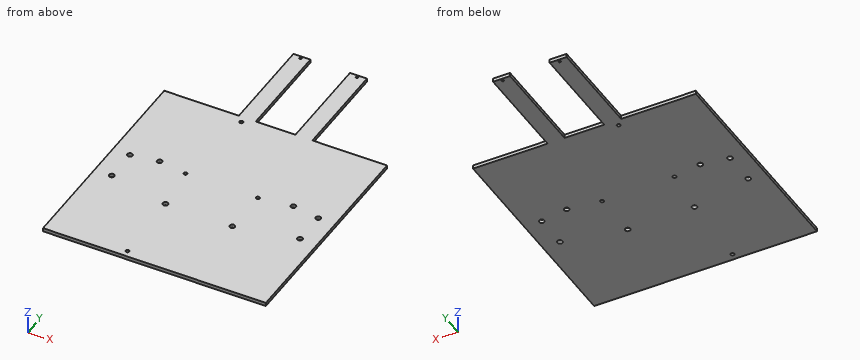
from build123d import *

# Parameters (mm, degrees)
F0_W     = 51.8
F0_H     = 10
F0_W_2   = 15.24
F0_H_2   = 34.925
F0_R     = 2.3114
F0_R_2   = 1.05
F0_R_3   = 1.5875
F0_W_3   = 9.38
F1_DEPTH = 3.175
F2_DEPTH = 90


# Not quite as in the source:
# - a length typed as a fraction of an inch, garbled in the dataset ("3 / 203.2 mm" for 3/8 in), is restored
# - a feature names something its author has since deleted; it is built from what else it names


with BuildPart() as f1:
    # F0 (on Top) → F1 (new body)
    with BuildSketch(Plane.XY):
        Polygon((42.4, -100), (100, -100), (100, -75.075), (48.2, -75.075), (48.2, -65.075), (33.02, -65.075), (33.02, -100), align=None)
        with Locations((74.1, -70.075)):
            Rectangle(F0_W, F0_H)
        Polygon((33.02, -140), (33.02, -100), (17.78, -100), (17.78, -140), (17.78, -190), (25.4, -190), (33.02, -190), align=None)
        with BuildLine():
            ThreePointArc((26.45, -187.7), (26.1424621202, -188.4424621202), (25.4, -188.75))
            ThreePointArc((25.4, -188.75), (24.6575378798, -186.9575378798), (26.45, -187.7))
        make_face(mode=Mode.SUBTRACT)
        with Locations((25.4, -82.5375)):
            Rectangle(F0_W_2, F0_H_2)
        with Locations((74.1, -60.075)):
            Rectangle(F0_W, F0_H)
        Polygon((0, -100), (17.78, -100), (17.78, -65.075), (-17.78, -65.075), (-17.78, -100), align=None)
        Polygon((17.78, -65.075), (33.02, -65.075), (48.2, -65.075), (48.2, -55.075), (-48.2, -55.075), (-48.2, -65.075), (-33.02, -65.075), (-17.78, -65.075), align=None)
        with BuildLine():
            Line((48.2, -55.075), (100, -55.075))
            Line((100, -55.075), (100, -26.575))
            Line((100, -26.575), (32.3114, -26.575))
            ThreePointArc((32.3114, -26.575), (30, -28.8864), (27.6886, -26.575))
            Line((27.6886, -26.575), (0, -26.575))
            Line((0, -26.575), (-27.6886, -26.575))
            ThreePointArc((-27.6886, -26.575), (-30, -28.8864), (-32.3114, -26.575))
            Line((-32.3114, -26.575), (-100, -26.575))
            Line((-100, -26.575), (-100, -55.075))
            Line((-100, -55.075), (-48.2, -55.075))
            Line((-48.2, -55.075), (48.2, -55.075))
        make_face()
        with BuildLine():
            Line((32.3114, -26.575), (100, -26.575))
            Line((100, -26.575), (100, 0))
            Line((100, 0), (0, 0))
            Line((0, 0), (0, -10.4469014332))
            Line((0, -10.4469014332), (0, -26.575))
            Line((0, -26.575), (27.6886, -26.575))
            ThreePointArc((27.6886, -26.575), (30, -24.2636), (32.3114, -26.575))
        make_face()
        with Locations((84.5, -15)):
            Circle(F0_R, mode=Mode.SUBTRACT)
        Polygon((-17.78, -140), (-17.78, -100), (-27.462, -100), (-33.02, -100), (-33.02, -140), (-33.02, -190), (-25.4, -190), (-17.78, -190), align=None)
        with BuildLine():
            ThreePointArc((-24.35, -187.7), (-24.6575378798, -188.4424621202), (-25.4, -188.75))
            ThreePointArc((-25.4, -188.75), (-26.1424621202, -186.9575378798), (-24.35, -187.7))
        make_face(mode=Mode.SUBTRACT)
        with Locations((-25.4, -137.7)):
            Circle(F0_R_2, mode=Mode.SUBTRACT)
        Polygon((-27.462, -100), (-17.78, -100), (-17.78, -65.075), (-33.02, -65.075), (-33.02, -100), align=None)
        with BuildLine():
            ThreePointArc((-25.8745, -93.912), (-26.3394679849, -95.0345320151), (-27.462, -95.4995))
            ThreePointArc((-27.462, -95.4995), (-29.0495, -93.912), (-27.462, -92.3245))
            ThreePointArc((-27.462, -92.3245), (-26.3394679849, -92.7894679849), (-25.8745, -93.912))
        make_face(mode=Mode.SUBTRACT)
        with BuildLine():
            Line((0, 0), (100, 0))
            Line((100, 0), (100, 55.075))
            Line((100, 55.075), (48.2, 55.075))
            Line((48.2, 55.075), (48.2, 65.075))
            Line((48.2, 65.075), (42.4, 65.075))
            Line((42.4, 65.075), (42.4, 18.9709383994))
            Line((42.4, 18.9709383994), (42.4, 9.75))
            Line((42.4, 9.75), (30.355, 9.75))
            Line((30.355, 9.75), (-42.4, 9.75))
            Line((-42.4, 9.75), (-42.4, 65.075))
            Line((-42.4, 65.075), (-48.2, 65.075))
            Line((-48.2, 65.075), (-48.2, 55.075))
            Line((-48.2, 55.075), (-100, 55.075))
            Line((-100, 55.075), (-100, 0))
            Line((-100, 0), (-100, -26.575))
            Line((-100, -26.575), (-32.3114, -26.575))
            ThreePointArc((-32.3114, -26.575), (-30, -24.2636), (-27.6886, -26.575))
            Line((-27.6886, -26.575), (0, -26.575))
            Line((0, -26.575), (0, -10.4469014332))
            Line((0, -10.4469014332), (0, 0))
        make_face()
        with BuildLine():
            ThreePointArc((-82.1886, -15), (-86.134406614, -16.634406614), (-84.5, -12.6886))
            ThreePointArc((-84.5, -12.6886), (-82.865593386, -13.365593386), (-82.1886, -15))
        make_face(mode=Mode.SUBTRACT)
        with BuildLine():
            ThreePointArc((-82.1886, 15), (-82.865593386, 13.365593386), (-84.5, 12.6886))
            ThreePointArc((-84.5, 12.6886), (-86.134406614, 16.634406614), (-82.1886, 15))
        make_face(mode=Mode.SUBTRACT)
        with Locations((-60, 18.9709383994)):
            Circle(F0_R, mode=Mode.SUBTRACT)
        with BuildLine():
            ThreePointArc((62.3114, 18.9709383994), (60, 16.6595383994), (57.6886, 18.9709383994))
            ThreePointArc((57.6886, 18.9709383994), (60, 21.2823383994), (62.3114, 18.9709383994))
        make_face(mode=Mode.SUBTRACT)
        with Locations((84.5, 15)):
            Circle(F0_R, mode=Mode.SUBTRACT)
        with Locations((-74.1, -60.075)):
            Rectangle(F0_W, F0_H)
        Polygon((-33.02, -100), (-33.02, -65.075), (-48.2, -65.075), (-48.2, -75.075), (-100, -75.075), (-100, -100), (-42.4, -100), align=None)
        with Locations((74.1, 60.075)):
            Rectangle(F0_W, F0_H)
        with Locations((-74.1, -70.075)):
            Rectangle(F0_W, F0_H)
        with Locations((74.1, 70.075)):
            Rectangle(F0_W, F0_H)
        Polygon((48.2, 75.075), (100, 75.075), (100, 100), (42.4, 100), (42.4, 65.075), (48.2, 65.075), align=None)
        Polygon((42.4, 18.9709383994), (42.4, 65.075), (42.4, 100), (33.02, 100), (17.78, 100), (0, 100), (-17.78, 100), (-27.462, 100), (-33.02, 100), (-33.02, 65.075), (-42.4, 65.075), (-42.4, 9.75), (30.355, 9.75), (42.4, 9.75), align=None)
        with Locations((-34.645, 14.954)):
            Circle(F0_R_3, mode=Mode.SUBTRACT)
        with BuildLine():
            ThreePointArc((-27.462, 92.3245), (-29.0495, 93.912), (-27.462, 95.4995))
            ThreePointArc((-27.462, 95.4995), (-26.3394679849, 95.0345320151), (-25.8745, 93.912))
            ThreePointArc((-25.8745, 93.912), (-26.3394679849, 92.7894679849), (-27.462, 92.3245))
        make_face(mode=Mode.SUBTRACT)
        with BuildLine():
            ThreePointArc((31.9425, 14.954), (31.4775320151, 13.8314679849), (30.355, 13.3665))
            ThreePointArc((30.355, 13.3665), (29.2324679849, 13.8314679849), (28.7675, 14.954))
            ThreePointArc((28.7675, 14.954), (30.355, 16.5415), (31.9425, 14.954))
        make_face(mode=Mode.SUBTRACT)
        with Locations((-74.1, 60.075)):
            Rectangle(F0_W, F0_H)
        with Locations((-74.1, 70.075)):
            Rectangle(F0_W, F0_H)
        Polygon((17.78, 100), (33.02, 100), (33.02, 140), (33.02, 190), (25.4, 190), (17.78, 190), (17.78, 140), align=None)
        with BuildLine():
            ThreePointArc((26.45, 187.7), (24.6575378798, 186.9575378798), (25.4, 188.75))
            ThreePointArc((25.4, 188.75), (26.1424621202, 188.4424621202), (26.45, 187.7))
        make_face(mode=Mode.SUBTRACT)
        Polygon((-100, 100), (-100, 75.075), (-48.2, 75.075), (-48.2, 65.075), (-42.4, 65.075), (-42.4, 100), align=None)
        with Locations((-37.71, 82.5375)):
            Rectangle(F0_W_3, F0_H_2)
        Polygon((-27.462, 100), (-17.78, 100), (-17.78, 140), (-17.78, 190), (-25.4, 190), (-33.02, 190), (-33.02, 140), (-33.02, 100), align=None)
        with BuildLine():
            ThreePointArc((-24.35, 187.7), (-26.1424621202, 186.9575378798), (-25.4, 188.75))
            ThreePointArc((-25.4, 188.75), (-24.6575378798, 188.4424621202), (-24.35, 187.7))
        make_face(mode=Mode.SUBTRACT)
        with Locations((-25.4, -137.7)):
            Circle(F0_R_2)
    extrude(amount=F1_DEPTH)

    # F2 (cut): faces of the model
    f2_faces = [f1.faces().sort_by_distance(p)[0] for p in [
        (25.4, -190, 1.5875),
        (-25.4, -190, 1.5875),
    ]]
    extrude(f2_faces, amount=-F2_DEPTH, mode=Mode.SUBTRACT)


solid = f1.part
The listing builds one solid part. Answer for the finished solid, in the listing's coordinates (mm). Coordinates: 2 decimals unless noted, no trailing zeros. Write each loop counter-clockwise with the first axis right and the second up, starting at its lowest first coordinate (ties: lowest second). Pieces come first, ordered by that corner, then holes. Notation, with made-up numbers: M 53.25,86 L 62.25,86 A23 cw 62.25,118 Z; hole C 82.25,-26.5 d6. An arc over 180 degrees is marked long. Put each result on its own line as item: value. Start each with the question number.
1. Consider line 1 (X direction, y = 187.7, z = 0.75); line 2 (Y direction, x = 84.5, z = 2.1); line 3 (X direction, y = -28.5, z = 2.3). Determine where each line is inside the solid, lowest interval first. Write a range as from..to.
2. Flat-ended cylindrical pins translate along their axes: P1, Ø3, axis at x = 84.5, y = 15, coming from the +Z side; P2, Ø2.5, axis at x = -25.4, y = 187.7, coming from the +Z side (3 decimals); P3, Ø1, axis at y = 148.5, z = 1, coming from the -X side. Find the tip coordinate at first contact, or state that the pin passes through.
3. A cutting plane is placed at C-C on z = 1.1. Count the separate pieces of the cut face and the enclosed holes in it, then the cut area to 3 significant figures.
4. A cutting plane is placed at B-B on x = -44. Write down the section's boundary in (y, z) (3 decimals).
5. A cutting plane is placed at A-A on y = 154. Write down the section's boundary in (x, z) (3 decimals).
Resolved:
1. line 1: x = -33.02..-26.45, -24.35..-17.78, 17.78..24.35, 26.45..33.02
1. line 2: y = -100..-17.31, -12.69..12.69, 17.31..100
1. line 3: x = -100..-31.28, -28.72..28.72, 31.28..100
2. P1: passes through
2. P2: stops at z = 3.175
2. P3: stops at x = -33.02
3. separate pieces: 1
3. enclosed holes: 14
3. area: 42,600 mm2
4. outline: M -100,0 L 100,0 L 100,3.175 L -100,3.175 Z
5. outline: M -33.02,0 L -17.78,0 L -17.78,3.175 L -33.02,3.175 Z; M 17.78,0 L 33.02,0 L 33.02,3.175 L 17.78,3.175 Z
